Input: part model. Units: mm. Frame: model coordinates. A direction names the side the tool comes from. Coordinates: 2 decimals unless noted, no trailing zeros. Order: outer loops, then holes, each group sorted by start corner. A loop starts at its lowest first (then second) coordinate and runs counter-clockwise, first axis right, second up. Notation, with made-up numbers: M 57.5,2.25 L 109.5,2.25 A19 ccw 109.5,6.25 Z; hole C 72.5,77.5 d9. An arc over 180 degrees is marked long. Answer in a Markdown table with one row per item.
from build123d import *

# Parameters (mm, degrees)
F0_W     = 120.528899
F0_H     = 120.2101
F1_DEPTH = 69.4
F2_R     = 5
F3_T     = -2.5


with BuildPart() as f1:
    # F0 (on Top) → F1 (new body)
    with BuildSketch(Plane.XY):
        with Locations((8.009833, -5.004426)):
            Rectangle(F0_W, F0_H)
    extrude(amount=F1_DEPTH)

    # F2
    f2_edges = [f1.edges().sort_by_distance(p)[0] for p in [
        (8.009832, -65.109476, 69.4),
        (68.274282, -5.004426, 69.4),
        (68.274282, -65.109476, 34.7),
    ]]
    fillet(f2_edges, radius=F2_R)

    # F3
    f3_openings = [f1.faces().sort_by_distance(p)[0] for p in [
        (7.987923, -4.982576, 0),
    ]]
    offset(amount=F3_T, openings=f3_openings)


solid = f1.part
1) Reachability of faces 4 (the face through (68.274, -3, 32)), 5 (the face through (7, 52.601, 33)) from +Z, -Z, +X, -X, +Y, -Y: full face, straight path, thin tool, end or side. Return the list, or none.
Resolved:
| item | result |
|---|---|
| face 4 | +Z, -Z, +X, +Y, -Y |
| face 5 | -Z |
2) Cut plane B-B, the plane y = 45.5. Output: boundary loops of the cut face in (x, z).
Resolved:
| item | result |
|---|---|
| outline | M -52.25,0 L -49.75,0 L -49.75,66.9 L 63.27,66.9 A2.5 cw 65.77,64.4 L 65.77,0 L 68.27,0 L 68.27,64.4 A5 ccw 63.27,69.4 L -52.25,69.4 Z |
3) Cut plane C-C, the plane x = 30. Output: boundary loops of the cut face in (y, z).
Resolved:
| item | result |
|---|---|
| outline | M -65.11,0 L -62.61,0 L -62.61,64.4 A2.5 cw -60.11,66.9 L 52.6,66.9 L 52.6,0 L 55.1,0 L 55.1,69.4 L -60.11,69.4 A5 ccw -65.11,64.4 Z |
4) Cut plane A-A, the plane z = 35.5. Output: boundary loops of the cut face in (x, y).
Resolved:
| item | result |
|---|---|
| outline | M -52.25,-65.11 L 63.27,-65.11 A5 ccw 68.27,-60.11 L 68.27,55.1 L -52.25,55.1 Z; hole M -49.75,-62.61 L 63.27,-62.61 A2.5 ccw 65.77,-60.11 L 65.77,52.6 L -49.75,52.6 Z |
5) Mould query, pull axis Y, two halves, no side actions, for faces 1 (the face through (-19, 53, 0)), 2 (the face through (66.771, -63.684, 32.651)), 3 (the face through (6, -3, 66.9)). Classes: +Y half, -Y half, draft (parallel to the pull), parting line (faces both ways), or undercut.
Resolved:
| item | result |
|---|---|
| face 1 | draft |
| face 2 | -Y half |
| face 3 | undercut |
6) Contact query for a flat-ended pin moving along its axis: pin 1 (1.5 mm diameter, centred on x = 39, y = -20.5, fed in from -Z). Output: stop coordinate, or through.
Resolved:
| item | result |
|---|---|
| pin 1 | stops at z = 66.9 |
7) Material intervals for probe 1 along Y at (x, z) = (-40.5, 11.5); probe 2 along X at (y, z) = (0, 19); probe 3 along Z at (x, y) = (22, -27), sorted ascending.
Resolved:
| item | result |
|---|---|
| probe 1 | y = -65.11 to -62.61, 52.6 to 55.1 |
| probe 2 | x = -52.25 to -49.75, 65.77 to 68.27 |
| probe 3 | z = 66.9 to 69.4 |
